Work out the finished part from the listing and answer in its coordinate system (mm). Give positions to 0.01 mm unless a question says otherwise; leave off trailing zeros. Loops run counter-clockwise (first coordinate to the right, second up) from the corner with the lowest first, then second, coordinate; pieces in that order, holes last. Notation, with made-up numbers: (68.5, 11) - (120.5, 11) arc R15 cw to (120.5, 29) - close; hole circle Ø4 at (73.5, -29.5). An arc over 180 degrees is marked (long way). One line per question, with ' | ' between items.
Autodesk Inventor part; units mm, degrees
ref_plane "YZ Plane" through (0, 0, 0) normal (1, 0, 0) x (0, 1, 0)
ref_plane "XZ Plane" through (0, 0, 0) normal (0, 1, 0) x (-1, 0, 0)
ref_plane "XY Plane" through (0, 0, 0) normal (0, 0, 1) x (1, 0, 0)
sketch "Sketch1" plane through (0, 0, 0) normal (0, 0, 1) x (1, 0, 0)
  circle A0 centre (0, 0) radius 2
  line L0 (-3.5, 3.5) -> (3.5, 3.5)
  line L1 (3.5, 3.5) -> (3.5, -3.5)
  line L2 (3.5, -3.5) -> (-3.5, -3.5)
  line L3 (-3.5, -3.5) -> (-3.5, 3.5)
  point P0 (3.5, 0)
  point P1 (0, 3.5)
  dimension "d0" = 4
  dimension "d24" = 7
extrude "Extrusion1" add sketch "Sketch1" along normal blind 3
fillet "Fillet3" radius 2 4 edges at (3.5, 3.5, 1.5) (3.5, -3.5, 1.5) (-3.5, -3.5, 1.5) (-3.5, 3.5, 1.5)
chamfer "Chamfer4" distance 0.4 angle 45 18 edges at (-2.9142, -2.9142, 3) (-3.5, 0, 3) (-2.9142, 2.9142, 3) (0, 3.5, 3) (2.9142, 2.9142, 3) (3.5, 0, 3) (2.9142, -2.9142, 3) (0, -3.5, 3) (2.9142, -2.9142, 0) (3.5, 0, 0) (2.9142, 2.9142, 0) (0, 3.5, 0) (-2.9142, 2.9142, 0) (-3.5, 0, 0) (-2.9142, -2.9142, 0) (0, -3.5, 0) (-2, 0, 3) (-2, 0, 0)
properties part number "shaft-10mm" material "ABS Plastic"
1. Determine the mould class of faces 1 (the conical face through (-2.725, -2.699, 0.114)), 2 (the conical face through (2.699, 2.725, 2.886)), 3 (the cylindrical face through (0, 2, 1)) for opening direction Y: +Y half, -Y half, draft (parallel to the pull), parting line (faces both ways), or undercut.
Evaluation:
face 1: -Y half | face 2: +Y half | face 3: undercut
2. Find section C-C on z = 1.2. Write down the section's boundary in (x, y), then the cut area to 3 significant figures.
Evaluation:
outline: (-3.5, -1.5) arc R2 ccw to (-1.5, -3.5) - (1.5, -3.5) arc R2 ccw to (3.5, -1.5) - (3.5, 1.5) arc R2 ccw to (1.5, 3.5) - (-1.5, 3.5) arc R2 ccw to (-3.5, 1.5) - close; hole circle Ø4 at (0, 0) | area: 33.0 mm2
3. Find section A-A on x = 0. Write down the section's boundary in (y, z), then the cut area to 3 significant figures.
Evaluation:
outline: (-3.5, 0.4) - (-3.1, 0) - (-2.4, 0) - (-2, 0.4) - (-2, 2.6) - (-2.4, 3) - (-3.1, 3) - (-3.5, 2.6) - close; (2, 0.4) - (2.4, 0) - (3.1, 0) - (3.5, 0.4) - (3.5, 2.6) - (3.1, 3) - (2.4, 3) - (2, 2.6) - close | area: 8.36 mm2
4. Consider L1, parallel to Y at x = 0, z = 1.4; L2, parallel to X at y = 1.5, z = 1.5; L3, parallel to X at y = 0.25, z = 0.35. Determine where each line is inside the solid, lowest interval first.
Evaluation:
L1: -3.5 to -2, 2 to 3.5 | L2: -3.5 to -1.32, 1.32 to 3.5 | L3: -3.45 to -2.03, 2.03 to 3.45
